from build123d import *

# Parameters (mm, degrees)
F0_R     = 12.5
F1_DEPTH = 2
F2_R     = 1.3161451829
F3_DEPTH = 25


with BuildPart() as f1:
    # F0 (on Top) → F1 (new body)
    with BuildSketch(Plane.XY):
        with BuildLine():
            ThreePointArc((15, -9.0138781887), (16.863421954, -4.6770717335), (17.5, 0))
            ThreePointArc((17.5, 0), (16.863421954, 4.6770717335), (15, 9.0138781887))
            Line((15, 9.0138781887), (15, -9.0138781887))
        make_face()
        with BuildLine():
            ThreePointArc((15, 9.0138781887), (16.863421954, 4.6770717335), (17.5, 0))
            ThreePointArc((17.5, 0), (16.863421954, -4.6770717335), (15, -9.0138781887))
            Line((15, -9.0138781887), (15, -17.5))
            Line((15, -17.5), (20, -17.5))
            Line((20, -17.5), (20, 17.5))
            Line((20, 17.5), (15, 17.5))
            Line((15, 17.5), (15, 9.0138781887))
        make_face()
        with BuildLine():
            Line((15, -9.0138781887), (15, 9.0138781887))
            ThreePointArc((15, 9.0138781887), (-17.5, 0), (15, -9.0138781887))
        make_face()
        Circle(F0_R, mode=Mode.SUBTRACT)
    extrude(amount=F1_DEPTH)

    # F2 (on face) → F3 (join)
    with BuildSketch(Plane.XY.offset(2)):
        with Locations((17.6118854433, 15.5552299693)):
            Circle(F2_R)
    extrude(amount=F3_DEPTH)


solid = f1.part
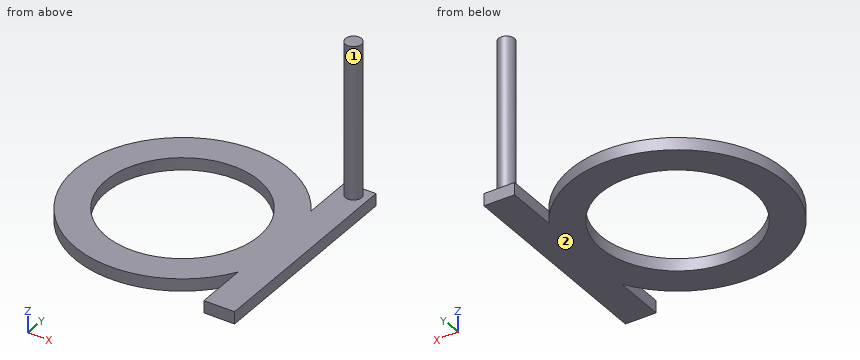
Geometry: final body of the model. Coordinates: model frame, mm. Face numbers are marked on the shaded views. A direction names the side the tool comes from. Round coordinates to 2 decimals unless told otherwise and drop trailing zeros. Loops run counter-clockwise (first coordinate to the right, second up) from the corner with the lowest first, then second, coordinate; pieces in that order, holes last. Notation, with made-up numbers: (38.25, 54.5) -> (60.25, 54.5) arc R29 ccw to (60.25, 83.5) -> close; hole circle Ø8 at (-37, 24.5). An arc over 180 degrees is marked (long way). One line per question, with ' | ' between items. Start each with the question number.
1. Contact query for flat-ended pins moving along their axis: pin 1 (15 mm diameter, centred on x = 0, y = 0, fed in from +Z); pin 2 (2 mm diameter, centred on y = -12, z = 1, fed in from -X); pin 3 (10.5 mm diameter, centred on x = -8, y = -4.5, fed in from +Z); pin 4 (0.6 mm diameter, centred on y = 12, z = 1.5, fed in from -X). Output: stop coordinate, or through.
2. Section A-A on y = 0. Output: boundary loops of the cut face in (x, z).
3. Section D-D on z = 22.5. Output: boundary loops of the cut face in (x, y), and give its area (3 significant figures).
4. Section C-C on x = -15. Output: boundary loops of the cut face in (y, z), and give its area (3 significant figures).
5. Set-up query: the marked faces 1 and 2. Return all of +Z, -Z, +X, -X, +Y, -Y with unobstructed straight access to the full face (end or side cutting, diameter ignored); none if empty.
6. Line query: line 1 along Y through (x, z) = (0, 0.55); line 2 along Z through (x, y) = (-3, -12.5); line 3 along Y through (x, z) = (-15.5, 1). Output: solid intervals per line, ascending. Write a range as [from, to].
7. Section B-B on x = 0. Output: boundary loops of the cut face in (y, z), and give its area (3 significant figures).
Returned:
1) pin 1: passes through | pin 2: stops at x = -13.61 | pin 3: stops at z = 2 | pin 4: stops at x = -13.01
2) outline: (-17.5, 0) -> (-12.5, 0) -> (-12.5, 2) -> (-17.5, 2) -> close; (12.5, 0) -> (20, 0) -> (20, 2) -> (12.5, 2) -> close
3) outline: circle Ø2.63 at (17.61, 15.56) | area: 5.44 mm2
4) outline: (-9.01, 0) -> (9.01, 0) -> (9.01, 2) -> (-9.01, 2) -> close | area: 36.1 mm2
5) face 1: +Z | face 2: -Z, +X, -X, +Y, -Y
6) line 1: y = [-17.5, -12.5], [12.5, 17.5] | line 2: z = [0, 2] | line 3: y = [-8.12, 8.12]
7) outline: (-17.5, 0) -> (-12.5, 0) -> (-12.5, 2) -> (-17.5, 2) -> close; (12.5, 0) -> (17.5, 0) -> (17.5, 2) -> (12.5, 2) -> close | area: 20.0 mm2
